Could you check a few things on this drawing? It's one solid part, dimensions in mm from its lowest x, y, z. Give positions to 0.01 mm unless a question says otherwise; leave off trailing zeros. Loops run counter-clockwise (first coordinate to the right, second up) from the corner with the lowest first, then second, coordinate; pieces in that order, holes last.
Q1. I need wall thicknesses on probe 1 along X at (y, z) = (5, 23); probe 2 along Y at (x, z) = (30, 3); probe 3 along X at (y, z) = (9, 21.5). Which ranges of each line are inside material? Lowest first, please.
Q2. I'm going to push flat-ended pins straight in: P1, Ø1.3, axis at x = 23.075, y = 1.7, coming from the +Z side; P2, Ø12, axis at x = 28, z = 21.5, coming from the -Y side; P3, Ø4, axis at x = 19, y = 17, coming from the -Z side; P4, Ø1.8, axis at x = 23.075, y = 1.7, coming from the -Z side. Where does each tip first touch, or does it pass through?
Q3. Suppose I cut it at A-A (y = 1.7). Count the separate pieces of the cut face and the enclosed holes in it, and give its area (3 significant figures).
Q4. Thinking about a two-plate mould opening in Z: for the marked faces 1, 2 and 3, which applies, pulls with the +Z half, pulls with the -Z half, needs draft (parallel to the pull), parting line crosses it, or undercut?
Q5. Suppose I cut it at D-D (y = 15). List the corners of the cut face in (x, z) for me (3 decimals), and give its area (3 significant figures).
Q6. Suppose I cut it at B-B (z = 39). List the corners of the cut face in (x, y) for me, and give its area (3 significant figures).
Q7. Suppose I cut it at C-C (x = 9). List the corners of the cut face in (y, z) for me, and give its area (3 significant figures).
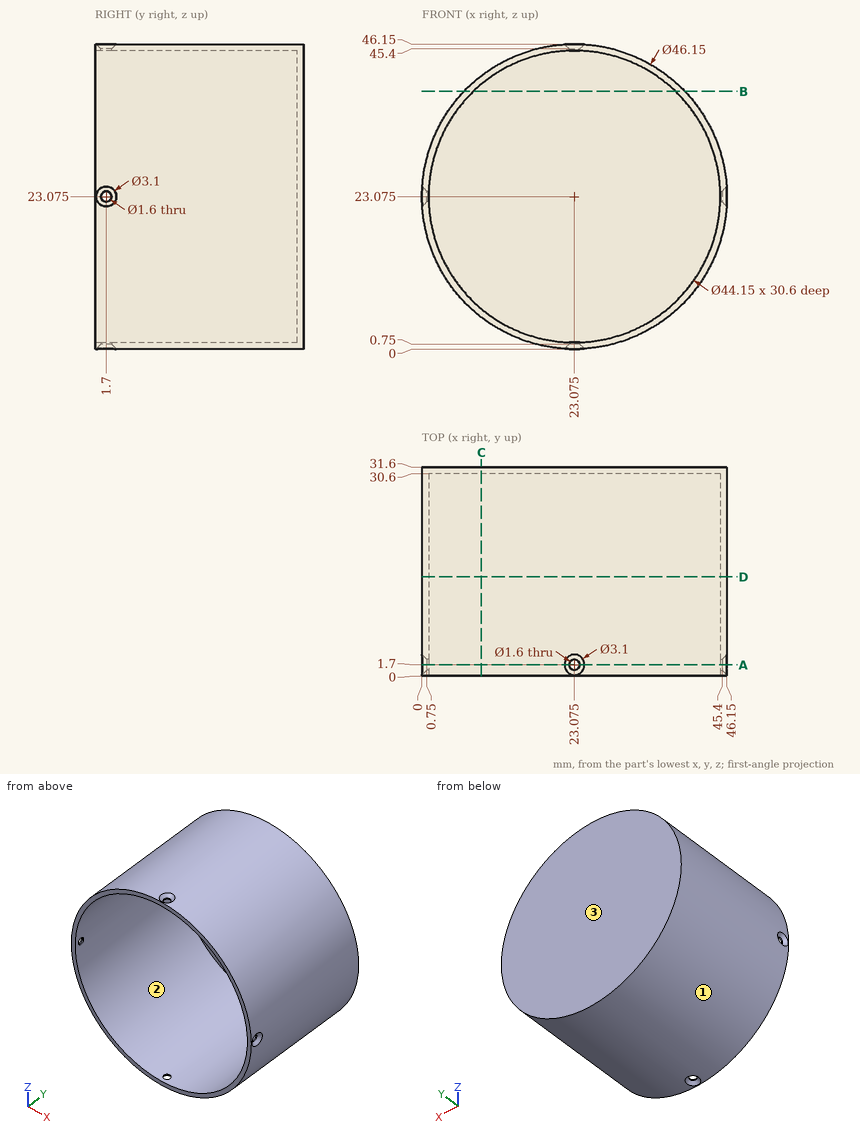
Solutions:
1. probe 1: x = 0 to 1, 45.15 to 46.15
1. probe 2: y = 30.6 to 31.6
1. probe 3: x = 0.05 to 1.06, 45.09 to 46.1
2. P1: passes through
2. P2: stops at y = 30.6
2. P3: stops at z = 0.09
2. P4: stops at z = 0.65
3. separate pieces: 4
3. enclosed holes: 0
3. area: 133 mm2
4. face 1: parting line crosses it
4. face 2: undercut
4. face 3: needs draft
5. outline: circle Ø46.15 at (23.075, 23.075); hole circle Ø44.15 at (23.075, 23.075)
5. area: 142 mm2
6. outline: (6.38, 0) - (7.79, 0) - (7.79, 30.6) - (38.36, 30.6) - (38.36, 0) - (39.77, 0) - (39.77, 31.6) - (6.38, 31.6) - close
6. area: 120 mm2
7. outline: (0, 4.79) - (31.6, 4.79) - (31.6, 41.36) - (0, 41.36) - (0, 40.08) - (30.6, 40.08) - (30.6, 6.07) - (0, 6.07) - close
7. area: 115 mm2
